The model under review builds one solid part; all positions refer to its coordinate system, in mm. Face numbers are marked on the shaded views. A direction names the side the tool comes from. Coordinates: 2 decimals unless noted, no trailing zeros. Order: outer loops, then holes, each group sorted by start corner. A loop starts at its lowest first (then second) coordinate and runs counter-clockwise, first axis right, second up. Notation, with made-up numbers: M 14,79 L 26,79 A13 cw 26,91 Z; hole C -37,-34.5 d9. An arc over 180 degrees is marked long. One line per item, written item: value.
```python
from build123d import *

# Parameters (mm, degrees)
F0_R     = 1.5
F1_DEPTH = 5.5
F0_R_2   = 2.5
F2_DEPTH = 1
F3_SIZE  = 0.5
F4_R     = 0.5
F5_DEPTH = 12.5


with BuildPart() as f1:
    # F0 (on Front) → F1 (new body)
    with BuildSketch(Plane.XZ):
        Circle(F0_R)
    extrude(amount=F1_DEPTH)

    # F0 (on Front) → F2 (join)
    with BuildSketch(Plane.XZ):
        Circle(F0_R_2)
        Circle(F0_R, mode=Mode.SUBTRACT)
        Circle(F0_R)
    extrude(amount=-F2_DEPTH)

    # F3
    f3_edges = [f1.edges().sort_by_distance(p)[0] for p in [
        (-1.5, -5.5, 0),
    ]]
    chamfer(f3_edges, length=F3_SIZE)

    # F4 (on Top) → F5 (cut, symmetric)
    with BuildSketch(Plane.XY):
        with Locations((0, -4)):
            Circle(F4_R)
    extrude(amount=F5_DEPTH, both=True, mode=Mode.SUBTRACT)


solid = f1.part
```
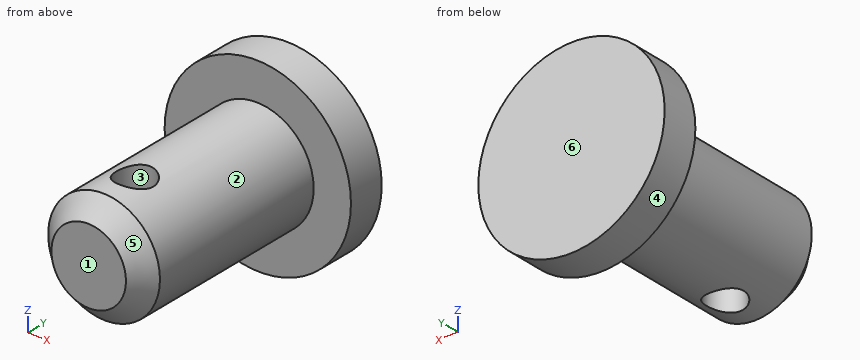
(1) Mouldability with a two-part tool opening along Y and no side actions: class the marked faces 3, 4, 5 and 6 as +Y half, -Y half, draft (parallel to the pull), parting line (faces both ways), or undercut.
Geometry results:
face 3: undercut
face 4: draft
face 5: -Y half
face 6: +Y half
(2) We need section C-C, the plane y = -3.75. State the section outline as (x, z) points.
Geometry results:
outline: M -0.43,-1.44 L -0.43,1.44 A1.5 ccw Z; M 0.43,-1.44 A1.5 ccw 0.43,1.44 Z
(3) We need section B-B, the plane z = 0. State the section outline as (x, y) points.
Geometry results:
outline: M -2.5,0 L -1.5,0 L -1.5,-5 L -1,-5.5 L 1,-5.5 L 1.5,-5 L 1.5,0 L 2.5,0 L 2.5,1 L -2.5,1 Z; hole C 0,-4 d1
(4) We need section D-D, the plane z = -2. State the section outline as (x, y) points.
Geometry results:
outline: M -1.5,0 L 1.5,0 L 1.5,1 L -1.5,1 Z
(5) We need section A-A, the plane x = 0. State the section outline as (y, z) points, plus the area to 4 significant figures.
Geometry results:
outline: M -5.5,-1 L -5,-1.5 L -4.5,-1.5 L -4.5,1.5 L -5,1.5 L -5.5,1 Z; M -3.5,-1.5 L 0,-1.5 L 0,-2.5 L 1,-2.5 L 1,2.5 L 0,2.5 L 0,1.5 L -3.5,1.5 Z
area: 18.25 mm2
(6) Insertion check: pin 1 Ø3 at (y, z) = (-4.5, 2) entering from +X. The pin has a flat end and moves straight along its axis. Give the tip position at first contact, or say it passes through.
Geometry results:
pin 1: stops at x = 1.41
(7) For L1, parallel to Y at x = 0, z = 0.1; L2, parallel to Y at x = 0, z = 1.8; L3, parallel to X at y = -4, z = 0.05, list the stretches that pass through material, from the lowest coordinate up.
Geometry results:
L1: y = -5.5 to -4.5, -3.5 to 1
L2: y = 0 to 1
L3: x = -1.5 to -0.5, 0.5 to 1.5
(8) Tool access review of the marked faces 1 and 2: name each direction out of +Z, -Z, +X, -X, +Y, -Y from which nothing blocks a thin tool from reaching the whole face with its end or side.
Geometry results:
face 1: +Z, -Z, +X, -X, -Y
face 2: -Y
